Here's how the part is built. I have some questions about the finished solid (model axes, mm). Give positions to 0.01 mm unless a question says otherwise; leave off trailing zeros. Loops run counter-clockwise (first coordinate to the right, second up) from the corner with the lowest first, then second, coordinate; pieces in that order, holes last.
Q1. If we section it at C-C (y = 95): Please give me the cut outline in (x, z).
Q2. If we section it at D-D (x = 45): Please give me the cut outline in (y, z).
Q3. I need wall thicknesses on line 1 (Y direction, x = 0, z = 2.6); line 2 (Y direction, x = -45, z = 2.5); line 3 (Y direction, x = 44.5, z = 1.65). Which ranges of each line are inside material? Lowest first, please.
Q4. If we section it at B-B (z = 1.2): Please give me the cut outline in (x, y).
Q5. If we section it at A-A (x = -45): Please give me the cut outline in (y, z), plus the area to 3 significant figures.
Q6. Will these pins go through, and if not, where does the flat tip stop? P1, Ø2, axis at y = 109.5, z = 2.5, coming from the -X side; P2, Ø2, axis at x = 25.5, z = 3.5, coming from the +Y side; P3, Ø2, axis at x = -43, z = 1, coming from the +Y side.
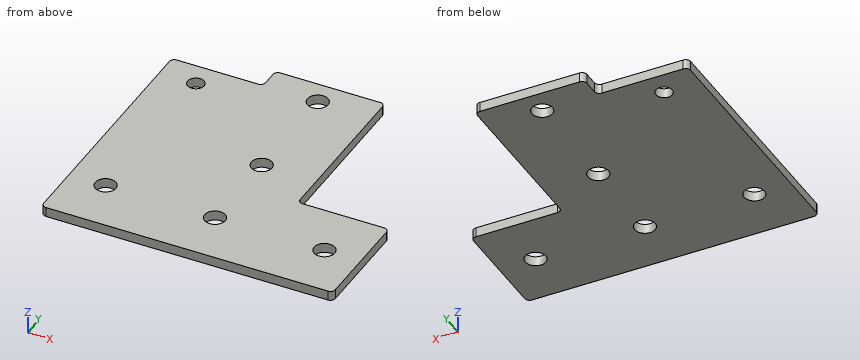
from build123d import *

# Parameters (mm, degrees)
SKETCH1_R           = 4.25
SKETCH1_R_2         = 3.4
BOSS_EXTRUDE1_DEPTH = 4
FILLET1_R           = 2


with BuildPart() as part:
    # Sketch1 → Boss-Extrude1 (new body)
    with BuildSketch(Plane.XY):
        Polygon((-60, 0), (60, 0), (60, 45), (22.5, 45), (22.5, 115), (-22.5, 115), (-22.5, 105), (-60, 105), (-60, 45), align=None)
        with Locations((0, 22.5)):
            Circle(SKETCH1_R, mode=Mode.SUBTRACT)
        with Locations((-45, 22.5)):
            Circle(SKETCH1_R, mode=Mode.SUBTRACT)
        with Locations((45, 22.5)):
            Circle(SKETCH1_R, mode=Mode.SUBTRACT)
        with Locations((0, 105)):
            Circle(SKETCH1_R, mode=Mode.SUBTRACT)
        with Locations((0, 60)):
            Circle(SKETCH1_R, mode=Mode.SUBTRACT)
        with Locations((-45, 95)):
            Circle(SKETCH1_R_2, mode=Mode.SUBTRACT)
    extrude(amount=BOSS_EXTRUDE1_DEPTH)

    # Fillet1
    fillet1_edges = [part.edges().sort_by_distance(p)[0] for p in [
        (-60, 105, 2),
        (-22.5, 105, 2),
        (-22.5, 115, 2),
        (22.5, 115, 2),
        (22.5, 45, 2),
        (60, 45, 2),
        (60, 0, 2),
        (-60, 0, 2),
    ]]
    fillet(fillet1_edges, radius=FILLET1_R)


solid = part.part
Check sheet entries:
1. outline: (-60, 0) - (-48.4, 0) - (-48.4, 4) - (-60, 4) - close; (-41.6, 0) - (22.5, 0) - (22.5, 4) - (-41.6, 4) - close
2. outline: (0, 0) - (18.25, 0) - (18.25, 4) - (0, 4) - close; (26.75, 0) - (45, 0) - (45, 4) - (26.75, 4) - close
3. line 1: y = 0 to 18.25, 26.75 to 55.75, 64.25 to 100.75, 109.25 to 115
3. line 2: y = 0 to 18.25, 26.75 to 91.6, 98.4 to 105
3. line 3: y = 0 to 18.28, 26.72 to 45
4. outline: (-60, 2) arc R2 ccw to (-58, 0) - (58, 0) arc R2 ccw to (60, 2) - (60, 43) arc R2 ccw to (58, 45) - (24.5, 45) arc R2 cw to (22.5, 47) - (22.5, 113) arc R2 ccw to (20.5, 115) - (-20.5, 115) arc R2 ccw to (-22.5, 113) - (-22.5, 107) arc R2 cw to (-24.5, 105) - (-58, 105) arc R2 ccw to (-60, 103) - close; hole circle Ø8.5 at (-45, 22.5); hole circle Ø6.8 at (-45, 95); hole circle Ø8.5 at (0, 22.5); hole circle Ø8.5 at (0, 60); hole circle Ø8.5 at (0, 105); hole circle Ø8.5 at (45, 22.5)
5. outline: (0, 0) - (18.25, 0) - (18.25, 4) - (0, 4) - close; (26.75, 0) - (91.6, 0) - (91.6, 4) - (26.75, 4) - close; (98.4, 0) - (105, 0) - (105, 4) - (98.4, 4) - close
5. area: 359 mm2
6. P1: stops at x = -22.5
6. P2: stops at y = 45
6. P3: stops at y = 105
